Work out the finished part from the listing and answer in its coordinate system (mm). A direction names the side the tool comes from. Coordinates: 2 decimals unless noted, no trailing zeros. Order: outer loops, then holes, each group sorted by start corner. A loop starts at its lowest first (then second) coordinate and runs counter-clockwise, first axis right, second up. Notation, with made-up numbers: (18.25, 62.5) -> (35.25, 62.5) arc R8 cw to (35.25, 73.5) -> close; hole circle Ø5 at (-33.5, -2). An arc over 180 degrees is marked (long way). Write item = value, one per line. Start each with the question number.
Q1. The part is cut by section C-C, the plane x = 28. Determine the outline of the cut face in (y, z), plus the area to 3 significant figures.
Q2. The part is cut by section B-B, the plane y = 18.5. Determine the outline of the cut face in (x, z), plus the area to 3 significant figures.
Q3. Which of the six approach directions +Z, -Z, +X, -X, +Y, -Y give full straight-line access (tool end or side, diameter ignored) to faces 4 (the cylindrical face through (51.3, -35.4, 32.5)), 5 (the flat face through (-53.75, 17, 33)), 6 (the cylindrical face through (40.88, 37.26, 56.3)), 7 (the cylindrical face through (-24.342, -37.26, 8.601))?
Q4. Flat-ended cylindrical pins translate along their axes: pin 1 (1.6 mm diameter, centred on x = 53, z = 23.5, fed in from -Y); pin 2 (0.8 mm diameter, centred on x = 53.5, z = 29.5, fed in from +Y); pin 3 (3 mm diameter, centred on y = -20.5, z = 52.5, fed in from +X). Find the tip coordinate at first contact, or state that the pin passes through.
Q5. The part is cut by section A-A, the plane z = 29. Count the separate pieces of the cut face and the enclosed holes in it, plus the area to 3 significant figures.
Q6. For a pull along Y with two mould halves and no side action, classify faces 1 (the cylindrical face through (-21.724, -37.26, 9.352)), 2 (the cylindrical face through (-65.7, -35.5, 32.5)), 3 (the cylindrical face through (53.01, -14.9, 8.86)) as +Y half, -Y half, draft (parallel to the pull), parting line (faces both ways), or undercut.
Q7. Straight lines are drawn through the part: L1, parallel to Z at x = -42, y = 37; L2, parallel to Y at x = 28, z = 11; L3, parallel to Z at x = 52.65, y = 9.5. For each, find the intervals that lie inside material, in ascending order. Write a range as from..to.
```python
from build123d import *

# Parameters (mm, degrees)
F1_DEPTH = 66
F2_R     = 2
F3_DEPTH = 25
F4_R     = 1.55
F5_DEPTH = 25
F6_R     = 1
F7_DEPTH = 25


# Not quite as in the source:
# - a feature names something its author has since deleted; it is built from what else it names


with BuildPart() as f1:
    # F0 (on Top) → F1 (new body)
    with BuildSketch(Plane.XY):
        with BuildLine():
            Line((-66.75, -33), (-66.75, 33))
            Line((-66.75, 33), (-68.25, 33))
            Line((-68.25, 33), (-68.25, -33))
            ThreePointArc((-68.25, -33), (-66.7855339059, -36.5355339059), (-63.25, -38))
            Line((-63.25, -38), (48.75, -38))
            ThreePointArc((48.75, -38), (52.2855339059, -36.5355339059), (53.75, -33))
            Line((53.75, -33), (53.75, 33))
            ThreePointArc((53.75, 33), (52.2855339059, 36.5355339059), (48.75, 38))
            Line((48.75, 38), (-48.75, 38))
            ThreePointArc((-48.75, 38), (-52.2855339059, 36.5355339059), (-53.75, 33))
            Line((-53.75, 33), (-53.75, 0))
            Line((-53.75, 0), (-52.25, 0))
            Line((-52.25, 0), (-52.25, 33))
            ThreePointArc((-52.25, 33), (-51.2248737342, 35.4748737342), (-48.75, 36.5))
            Line((-48.75, 36.5), (48.75, 36.5))
            ThreePointArc((48.75, 36.5), (51.2248737342, 35.4748737342), (52.25, 33))
            Line((52.25, 33), (52.25, -33))
            ThreePointArc((52.25, -33), (51.2248737342, -35.4748737342), (48.75, -36.5))
            Line((48.75, -36.5), (-63.25, -36.5))
            ThreePointArc((-63.25, -36.5), (-65.7248737342, -35.4748737342), (-66.75, -33))
        make_face()
    extrude(amount=F1_DEPTH)

    # F2 (on face) → F3 (cut)
    with BuildSketch(Plane.XZ.offset(38)):
        with BuildLine():
            Line((20.75, 52), (-23.25, 52))
            ThreePointArc((-23.25, 52), (-25.3713203436, 51.1213203436), (-26.25, 49))
            Line((-26.25, 49), (-26.25, 17))
            ThreePointArc((-26.25, 17), (-25.3713203436, 14.8786796564), (-23.25, 14))
            Line((-23.25, 14), (20.75, 14))
            ThreePointArc((20.75, 14), (22.8713203436, 14.8786796564), (23.75, 17))
            Line((23.75, 17), (23.75, 49))
            ThreePointArc((23.75, 49), (22.8713203436, 51.1213203436), (20.75, 52))
        make_face()
        with Locations((-26.25, 58)):
            Circle(F2_R)
        with Locations((23.75, 58)):
            Circle(F2_R)
        with Locations((23.75, 8)):
            Circle(F2_R)
        with Locations((-26.25, 8)):
            Circle(F2_R)
        with BuildLine():
            ThreePointArc((-8.75, 8.5), (-8.3106601718, 7.4393398282), (-7.25, 7))
            Line((-7.25, 7), (4.75, 7))
            ThreePointArc((4.75, 7), (5.8106601718, 7.4393398282), (6.25, 8.5))
            ThreePointArc((6.25, 8.5), (5.8106601718, 9.5606601718), (4.75, 10))
            Line((4.75, 10), (-7.25, 10))
            ThreePointArc((-7.25, 10), (-8.3106601718, 9.5606601718), (-8.75, 8.5))
        make_face()
        with Locations((-20.25, 8)):
            Circle(F2_R)
        with Locations((-20.25, 58)):
            Circle(F2_R)
        with Locations((17.75, 58)):
            Circle(F2_R)
        with Locations((14.75, 8)):
            Circle(F2_R)
    extrude(amount=-F3_DEPTH, mode=Mode.SUBTRACT)

    # F4 (on face) → F5 (cut)
    with BuildSketch(Plane(origin=(0, 38, 0), x_dir=(-1, 0, 0), z_dir=(0, 1, 0))):
        with Locations((-39.74, 55.25)):
            Circle(F4_R)
        with Locations((-39.74, 8)):
            Circle(F4_R)
        with Locations((42.25, 8.5)):
            Circle(F4_R)
        with Locations((42.25, 55.75)):
            Circle(F4_R)
        with Locations((42.25, 16.5)):
            Circle(F4_R)
        with Locations((42.25, 49.5)):
            Circle(F4_R)
    extrude(amount=-F5_DEPTH, mode=Mode.SUBTRACT)

    # F6 (on face) → F7 (cut)
    with BuildSketch(Plane.YZ.offset(53.75)):
        with BuildLine():
            Line((-17, 58), (-21, 58))
            ThreePointArc((-21, 58), (-23.1213203436, 57.1213203436), (-24, 55))
            Line((-24, 55), (-24, 11))
            ThreePointArc((-24, 11), (-23.1213203436, 8.8786796564), (-21, 8))
            Line((-21, 8), (-17, 8))
            ThreePointArc((-17, 8), (-14.8786796564, 8.8786796564), (-14, 11))
            Line((-14, 11), (-14, 55))
            ThreePointArc((-14, 55), (-14.8786796564, 57.1213203436), (-17, 58))
        make_face()
        with BuildLine():
            Line((24, 58), (-5, 58))
            ThreePointArc((-5, 58), (-7.1213203436, 57.1213203436), (-8, 55))
            Line((-8, 55), (-8, 11))
            ThreePointArc((-8, 11), (-7.1213203436, 8.8786796564), (-5, 8))
            Line((-5, 8), (24, 8))
            ThreePointArc((24, 8), (26.1213203436, 8.8786796564), (27, 11))
            Line((27, 11), (27, 55))
            ThreePointArc((27, 55), (26.1213203436, 57.1213203436), (24, 58))
        make_face()
        with Locations((-19, 61)):
            Circle(F6_R)
        with Locations((9.5, 61)):
            Circle(F6_R)
        with Locations((9.5, 5)):
            Circle(F6_R)
        with Locations((-19, 5)):
            Circle(F6_R)
    extrude(amount=-F7_DEPTH, mode=Mode.SUBTRACT)


solid = f1.part
```
Model answer:
q1.outline = (-38, 0) -> (-36.5, 0) -> (-36.5, 66) -> (-38, 66) -> close; (36.5, 0) -> (38, 0) -> (38, 66) -> (36.5, 66) -> close
q1.area = 198 mm2
q2.outline = (-68.25, 0) -> (-66.75, 0) -> (-66.75, 66) -> (-68.25, 66) -> close; (-53.75, 0) -> (-52.25, 0) -> (-52.25, 66) -> (-53.75, 66) -> close; (52.25, 0) -> (53.75, 0) -> (53.75, 8) -> (52.25, 8) -> close; (52.25, 58) -> (53.75, 58) -> (53.75, 66) -> (52.25, 66) -> close
q2.area = 222 mm2
q3.face_4 = +Z, -Z
q3.face_5 = +Z, -Z, +Y
q3.face_6 = +Y
q3.face_7 = -Y
q4.pin_1 = -36.62
q4.pin_2 = 35.47
q4.pin_3 = -66.75
q5.separate_pieces = 4
q5.enclosed_holes = 0
q5.area = 459 mm2
q6.face_1 = draft
q6.face_2 = +Y half
q6.face_3 = undercut
q7.L1 = 0..6.97, 10.03..14.97, 18.03..47.97, 51.03..54.22, 57.28..66
q7.L2 = -38..-36.5, 36.5..38
q7.L3 = 0..4, 6..8, 58..60, 62..66
